Design review of the part built by this model. Coordinates are the model's own, in mm. Face numbers are marked on the shaded views. A direction names the side the tool comes from. Give positions to 0.01 mm unless a question says otherwise; leave off trailing zeros. Loops run counter-clockwise (first coordinate to the right, second up) from the corner with the lowest first, then second, coordinate; pieces in that order, holes last. Notation, with made-up numbers: (18.5, 43.5) -> (50.5, 43.5) arc R30 cw to (50.5, 70.5) -> close; hole circle Ø8 at (3.5, -17.5). An arc over 180 degrees is marked (long way). Answer in a Markdown table with one row per item. Add a question column.
(1) Consider section D-D on z = 0. Count the separate pieces of the cut face and the enclosed holes in it, then the cut area to 3 significant figures.
(2) For pin 1 (5.5 mm diameter, centred on x = -15, y = 13, fed in from +Z); pin 2 (1 mm diameter, centred on y = 11.5, z = -3.5, fed in from +X); pin 3 (4 mm diameter, centred on x = -15, y = -5, fed in from -Z), all flat-tipped, find the tip position at first contact; note any pin that passes through.
(3) For the marked faces 4, 5 and 6, list the 3-axis set-ups (+Z, -Z, +X, -X, +Y, -Y) from which the entire face can be reached by the end or side of a thin tool; tool diameter is ignored.
(4) Consider section B-B on x = 15. Write out the cut boundary in (y, z), then the cut area to 3 significant figures.
(5) Draft analysis for pull direction X (two halves, no side actions). For the marked faces 1, 2 and 3, state which applies: +X half, -X half, draft (parallel to the pull), parting line (faces both ways), or undercut.
(6) For line 1 (Y direction, x = -15, z = 11); line 2 (X direction, y = -13, z = 11.5); line 3 (X direction, y = -13, z = 6.75), list the stretches that pass through material, from the lowest coordinate up.
from build123d import *

# Parameters (mm, degrees)
SKETCH_R        = 10.5
PAD_DEPTH       = 18
SKETCH002_R     = 2.5
POCKET_DEPTH    = 12
SKETCH003_R     = 2.15
POCKET001_DEPTH = 24.001
CHAMFER_SIZE    = 0.75
CHAMFER001_SIZE = 0.75
FILLET_R        = 0.5


with BuildPart() as casing_fillet:
    # Sketch → Pad (new body, symmetric)
    with BuildSketch(Plane.XZ):
        Polygon((-20, -9), (-20, 6), (-21, 7.6), (-21, 14), (-20, 15), (-10, 15), (-9, 14), (9, 14), (10, 15), (20, 15), (21, 14), (21, 7.6), (20, 6), (20, -9), (11, -9), (6, -13), (-6, -13), (-11, -9), align=None)
        Circle(SKETCH_R, mode=Mode.SUBTRACT)
    extrude(amount=PAD_DEPTH, both=True)

    # Sketch002 → Pocket (cut)
    with BuildSketch(Plane(origin=(0, 0, 15), x_dir=(-1, 0, 0), z_dir=(0, 0, 1))):
        with Locations((-15, 13)):
            Circle(SKETCH002_R)
        with Locations((15, 13)):
            Circle(SKETCH002_R)
        with Locations((-15, -13)):
            Circle(SKETCH002_R)
        with Locations((15, -13)):
            Circle(SKETCH002_R)
    extrude(amount=-POCKET_DEPTH, mode=Mode.SUBTRACT)

    # Sketch003 → Pocket001 (cut, through all)
    with BuildSketch(Plane(origin=(0, 0, -9), x_dir=(1, 0, 0), z_dir=(0, 0, -1))):
        with Locations((-15, 13)):
            Circle(SKETCH003_R)
        with Locations((15, 13)):
            Circle(SKETCH003_R)
        with Locations((15, -13)):
            Circle(SKETCH003_R)
        with Locations((-15, -13)):
            Circle(SKETCH003_R)
    extrude(amount=-POCKET001_DEPTH, mode=Mode.SUBTRACT)

    # Chamfer
    chamfer_edges = [casing_fillet.edges().sort_by_distance(p)[0] for p in [
        (-12.5, -13, 15),
        (-12.5, 13, 15),
        (17.5, 13, 15),
        (17.5, -13, 15),
    ]]
    chamfer(chamfer_edges, length=CHAMFER_SIZE)

    # Chamfer001
    chamfer001_edges = [casing_fillet.edges().sort_by_distance(p)[0] for p in [
        (12.85, 13, -9),
        (-17.15, 13, -9),
        (-17.15, -13, -9),
        (12.85, -13, -9),
    ]]
    chamfer(chamfer001_edges, length=CHAMFER001_SIZE)

    # Fillet
    fillet_edges = [casing_fillet.edges().sort_by_distance(p)[0] for p in [
        (-9, 0, 14),
        (9, 0, 14),
        (21, 0, 14),
        (20, 0, -9),
        (6, 0, -13),
        (11, 0, -9),
        (-6, 0, -13),
        (-11, 0, -9),
        (-20, 0, -9),
        (-21, 0, 14),
    ]]
    fillet(fillet_edges, radius=FILLET_R)


with BuildPart() as obj1:
    # Sketch001 → Revolution (revolve)
    with BuildSketch(Plane.YZ):
        Polygon((-15, 11), (15, 11), (15, 10), (14.5, 10), (14.5, 6.75), (15, 6.75), (15, 6), (-15, 6), (-15, 6.75), (-14.5, 6.75), (-14.5, 10), (-15, 10), align=None)
    revolve(axis=Axis((0, 0, 0), (0, 1, 0)))

    # Fusion: union casing-fillet
    add(casing_fillet.part)


solid = obj1.part
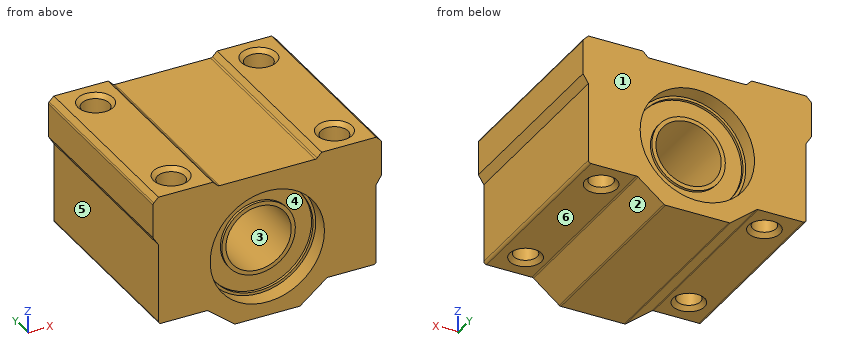
Values follow:
| question | item | result |
|---|---|---|
| 1 | separate pieces | 2 |
| 1 | enclosed holes | 4 |
| 1 | area | 889 mm2 |
| 2 | pin 1 | z = 14.5 |
| 2 | pin 2 | x = 20 |
| 2 | pin 3 | z = -9 |
| 3 | face 4 | -Y |
| 3 | face 5 | -Z, -X, +Y, -Y |
| 3 | face 6 | -Z, +X, +Y, -Y |
| 4 | outline | (-18, -9) -> (-15.9, -9) -> (-15.15, -8.25) -> (-15.15, 3) -> (-15.5, 3) -> (-15.5, 14.25) -> (-16.25, 15) -> (-18, 15) -> close; (-10.85, -8.25) -> (-10.1, -9) -> (10.1, -9) -> (10.85, -8.25) -> (10.85, 3) -> (10.5, 3) -> (10.5, 14.25) -> (9.75, 15) -> (-9.75, 15) -> (-10.5, 14.25) -> (-10.5, 3) -> (-10.85, 3) -> close; (15.15, -8.25) -> (15.9, -9) -> (18, -9) -> (18, 15) -> (16.25, 15) -> (15.5, 14.25) -> (15.5, 3) -> (15.15, 3) -> close |
| 4 | area | 639 mm2 |
| 5 | face 1 | draft |
| 5 | face 2 | +X half |
| 5 | face 3 | undercut |
| 6 | line 1 | -18 to -15.5, -10.5 to 10.5, 15.5 to 18 |
| 6 | line 2 | -21 to -17.5, -12.5 to 12.5, 17.5 to 21 |
| 6 | line 3 | -20.47 to -17.5, -12.5 to 12.5, 17.5 to 20.47 |
